from build123d import *

# Parameters (mm, degrees)
SKETCH1_W           = 350
SKETCH1_H           = 60
BOSS_EXTRUDE1_DEPTH = 15
SKETCH3_W           = 350
SKETCH3_H           = 15
BOSS_EXTRUDE4_DEPTH = 80
SKETCH5_W           = 350
SKETCH5_H           = 15
BOSS_EXTRUDE5_DEPTH = 90


with BuildPart() as part:
    # Sketch1 → Boss-Extrude1 (new body)
    with BuildSketch(Plane(origin=(0, 0, 0), x_dir=(1, 0, 0), z_dir=(0, 1, 0))):
        with Locations((175, -30)):
            Rectangle(SKETCH1_W, SKETCH1_H)
    extrude(amount=BOSS_EXTRUDE1_DEPTH)

    # Sketch3 → Boss-Extrude4 (add)
    with BuildSketch(Plane(origin=(0, 0, 0), x_dir=(-1, 0, 0), z_dir=(0, 0, -1))):
        with Locations((-175, 7.5)):
            Rectangle(SKETCH3_W, SKETCH3_H)
    extrude(amount=BOSS_EXTRUDE4_DEPTH)

    # Sketch5 → Boss-Extrude5 (add)
    with BuildSketch(Plane.XZ):
        with Locations((175, -72.5)):
            Rectangle(SKETCH5_W, SKETCH5_H)
    extrude(amount=BOSS_EXTRUDE5_DEPTH)


solid = part.part
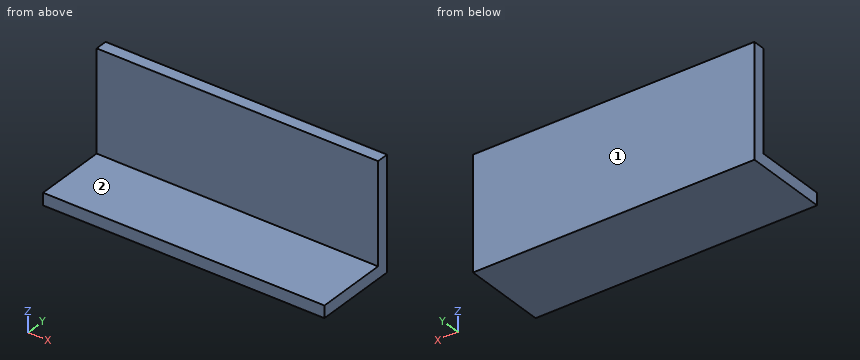
Read the model definition and answer for the solid it produces. Units are mm, in the model's axes. Face numbers are marked on the shaded views. A direction names the side the tool comes from. Coordinates: 2 decimals unless noted, no trailing zeros. Loops run counter-clockwise (first coordinate to the right, second up) from the corner with the lowest first, then second, coordinate; pieces in that order, holes last. Notation, with made-up numbers: (31, 31.5) -> (76, 31.5) arc R20 ccw to (76, 64.5) -> close; hole circle Ø2 at (67.25, 83). An arc over 180 degrees is marked (long way). Answer in a Markdown table with one row per item.
Item 1: Straight lines are drawn through the part: line 1 along Y through (x, z) = (201.5, -12.5); line 2 along Z through (x, y) = (131, -23). For each, find the intervals that lie inside material, in ascending order. Write a range as [from, to].
Returned:
| item | result |
|---|---|
| line 1 | y = [0, 15] |
| line 2 | z = [-80, -65] |
Item 2: For the marked faces 1 and 2, determine the directions among +Z, -Z, +X, -X, +Y, -Y from which every point of the face is accessible in a straight line to the end or side of a thin tool.
Returned:
| item | result |
|---|---|
| face 1 | +Z, -Z, +X, -X, +Y |
| face 2 | +Z, +X, -X, -Y |
Item 3: A cutting plane is placed at B-B on z = 16. Determine the outline of the cut face in (x, y), plus the area to 3 significant figures.
Returned:
| item | result |
|---|---|
| outline | (0, 0) -> (350, 0) -> (350, 15) -> (0, 15) -> close |
| area | 5,250 mm^2 |
Item 4: A cutting plane is placed at C-C on y = -83. Determine the outline of the cut face in (x, z).
Returned:
| item | result |
|---|---|
| outline | (0, -80) -> (350, -80) -> (350, -65) -> (0, -65) -> close |
Item 5: This flat-tipped pin is pushed along its axis until it touches: P1, Ø12, axis at x = 172.5, y = -14.5, coming from the +Z side. Where does it stop, or does it pass through?
Returned:
| item | result |
|---|---|
| P1 | stops at z = -65 |
Item 6: A cutting plane is placed at A-A on x = 315. Determine the outline of the cut face in (y, z), plus the area to 3 significant figures.
Returned:
| item | result |
|---|---|
| outline | (-90, -80) -> (15, -80) -> (15, 60) -> (0, 60) -> (0, -65) -> (-90, -65) -> close |
| area | 3,450 mm^2 |
